Check sheet for the modelled part. Datum: model origin and axes. Units: mm. Round coordinates to 2 decimals unless told otherwise and drop trailing zeros. Loops run counter-clockwise (first coordinate to the right, second up) from the corner with the lowest first, then second, coordinate; pieces in that order, holes last. Notation, with made-up numbers: (66.25, 6) - (81.25, 6) arc R22 cw to (81.25, 36) - close; hole circle Ø3 at (-18.5, -17.5). An arc over 180 degrees is marked (long way). Put each result on its own line as item: value. Start each with the question number.
```python
from build123d import *

# Parameters (mm, degrees)
SKETCH1_W           = 1866.9
SKETCH1_H           = 1219.2
BOSS_EXTRUDE1_DEPTH = 5.953125
SKETCH4_W           = 146.05
SKETCH4_H           = 95.25
CUT_EXTRUDE3_DEPTH  = 12.90625


with BuildPart() as part:
    # Sketch1 → Boss-Extrude1 (new body, symmetric)
    with BuildSketch(Plane(origin=(0, 0, 0), x_dir=(1, 0, 0), z_dir=(0, 1, 0))):
        Rectangle(SKETCH1_W, SKETCH1_H)
    extrude(amount=BOSS_EXTRUDE1_DEPTH, both=True)

    # Sketch4 → Cut-Extrude3 (cut, through all)
    with BuildSketch(Plane.XZ.offset(5.953125)):
        with Locations((352.425, -485.775)):
            Rectangle(SKETCH4_W, SKETCH4_H)
        with Locations((-352.425, -485.775)):
            Rectangle(SKETCH4_W, SKETCH4_H)
        with Locations((-606.425, 206.375)):
            Rectangle(SKETCH4_W, SKETCH4_H)
        with Locations((606.425, 206.375)):
            Rectangle(SKETCH4_W, SKETCH4_H)
    extrude(amount=-CUT_EXTRUDE3_DEPTH, mode=Mode.SUBTRACT)


solid = part.part
```
Q1. Cross-section at C-C on y = 2. Enter the section's corners in (x, z), and give its area (3 significant figures).
Q2. Cross-section at A-A on z = -464.5. Enter the section's corners in (x, y), and give its area (4 significant figures).
Q3. Material ranges on line 1 (X direction, y = 0.5, z = -507); line 2 (Z direction, x = 405.5, y = -1.25), recorded low to high. Write a range as from..to.
Q4. Cross-section at B-B on x = -600. Enter the section's corners in (y, z), and give its area (3 significant figures).
Answer list:
1. outline: (-933.45, -609.6) - (933.45, -609.6) - (933.45, 609.6) - (-933.45, 609.6) - close; hole (-679.45, 158.75) - (-533.4, 158.75) - (-533.4, 254) - (-679.45, 254) - close; hole (-425.45, -533.4) - (-279.4, -533.4) - (-279.4, -438.15) - (-425.45, -438.15) - close; hole (279.4, -533.4) - (425.45, -533.4) - (425.45, -438.15) - (279.4, -438.15) - close; hole (533.4, 158.75) - (679.45, 158.75) - (679.45, 254) - (533.4, 254) - close
1. area: 2,220,000 mm2
2. outline: (-933.45, -5.95) - (-425.45, -5.95) - (-425.45, 5.95) - (-933.45, 5.95) - close; (-279.4, -5.95) - (279.4, -5.95) - (279.4, 5.95) - (-279.4, 5.95) - close; (425.45, -5.95) - (933.45, -5.95) - (933.45, 5.95) - (425.45, 5.95) - close
2. area: 18,750 mm2
3. line 1: x = -933.45..-425.45, -279.4..279.4, 425.45..933.45
3. line 2: z = -609.6..-533.4, -438.15..609.6
4. outline: (-5.95, -609.6) - (5.95, -609.6) - (5.95, 158.75) - (-5.95, 158.75) - close; (-5.95, 254) - (5.95, 254) - (5.95, 609.6) - (-5.95, 609.6) - close
4. area: 13,400 mm2
